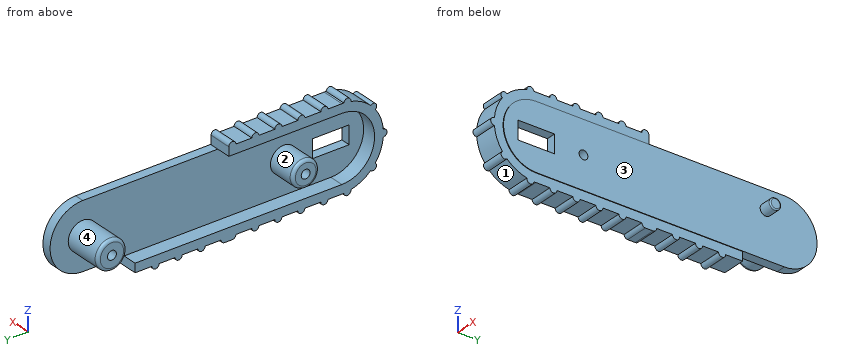
from build123d import *

# Parameters (mm, degrees)
PAD098_DEPTH            = 1.6
PAD099_DEPTH            = 4.05
POCKET093_DEPTH         = 0.1
SKETCH189_R             = 0.75
SKETCH189_W             = 6
SKETCH189_H             = 3
POCKET094_DEPTH         = 1.6
PAD100_DEPTH            = 3.95
SKETCH191_R             = 2.25
PAD101_DEPTH            = 4.9
SKETCH192_R             = 0.75
POCKET095_DEPTH         = 4.9
SKETCH193_R             = 2.475
PAD102_DEPTH            = 6.5
SKETCH194_R             = 0.75
POCKET096_DEPTH         = 6.5
FILLET041_R             = 0.5
SKETCH195_R             = 0.95
PAD103_DEPTH            = 2.2
FILLET042_R             = 0.2
SKETCH355_W             = 6.2
SKETCH355_H             = 3.1
POCKET171_DEPTH         = 5
BODY015_ROLL_ANGLE      = -90
BODY015_PLACEMENT_ANGLE = 90


with BuildPart() as part:
    # Sketch187 → Pad098 (new body)
    with BuildSketch(Plane.XY):
        with BuildLine():
            Line((0, 5.55), (42.05, 5.55))
            ThreePointArc((42.049962, -5.55), (47.599981, -1.9e-05), (42.05, 5.55))
            Line((42.049962, -5.55), (0, -5.55))
            ThreePointArc((0, 5.55), (-5.55, 0), (0, -5.55))
        make_face()
    extrude(amount=PAD098_DEPTH)

    # Sketch188 (on Face5 of Pad098) → Pad099 (join)
    with BuildSketch(Plane(origin=(0, 0, 0), x_dir=(1, 0, 0), z_dir=(0, 0, -1))):
        with BuildLine():
            Line((19.17, 5.55), (0, 5.55))
            ThreePointArc((0, 5.55), (-5.55, 0), (0, -5.55))
            Line((0, -5.55), (35.05, -5.55))
            Line((35.05, -5.55), (35.05, -7.05))
            Line((0, -7.05), (35.05, -7.05))
            ThreePointArc((0, 7.05), (-7.05, 0), (0, -7.05))
            Line((19.17, 7.05), (0, 7.05))
            Line((19.17, 5.55), (19.17, 7.05))
        make_face()
    extrude(amount=-PAD099_DEPTH)

    # Sketch188 (on Face5 of Pad098) → Pocket093 (cut)
    with BuildSketch(Plane(origin=(0, 0, 0), x_dir=(1, 0, 0), z_dir=(0, 0, -1))):
        with BuildLine():
            Line((19.17, 5.55), (0, 5.55))
            ThreePointArc((0, 5.55), (-5.55, 0), (0, -5.55))
            Line((0, -5.55), (35.05, -5.55))
            Line((35.05, -5.55), (35.05, -7.05))
            Line((0, -7.05), (35.05, -7.05))
            ThreePointArc((0, 7.05), (-7.05, 0), (0, -7.05))
            Line((19.17, 7.05), (0, 7.05))
            Line((19.17, 5.55), (19.17, 7.05))
        make_face()
    extrude(amount=-POCKET093_DEPTH, mode=Mode.SUBTRACT)

    # Sketch189 (on Face1 of Pocket093) → Pocket094 (cut)
    with BuildSketch(Plane(origin=(0, 0, 0), x_dir=(1, 0, 0), z_dir=(0, 0, -1))):
        with Locations((8, 0)):
            Circle(SKETCH189_R)
        Rectangle(SKETCH189_W, SKETCH189_H)
    extrude(amount=-POCKET094_DEPTH, mode=Mode.SUBTRACT)

    # Sketch190 (on Face11 of Pocket094) → Pad100 (join)
    with BuildSketch(Plane(origin=(0, 0, 0.1), x_dir=(1, 0, 0), z_dir=(0, 0, -1))):
        with BuildLine():
            ThreePointArc((19.17, 7.05), (18.57, 7.65), (17.97, 7.05))
            Line((19.17, 7.05), (17.97, 7.05))
        make_face()
        with BuildLine():
            ThreePointArc((15.27, 7.05), (14.67, 7.65), (14.07, 7.05))
            Line((15.27, 7.05), (14.07, 7.05))
        make_face()
        with BuildLine():
            ThreePointArc((11.37, 7.05), (10.77, 7.65), (10.17, 7.05))
            Line((11.37, 7.05), (10.17, 7.05))
        make_face()
        with BuildLine():
            ThreePointArc((7.47, 7.05), (6.87, 7.65), (6.27, 7.05))
            Line((7.47, 7.05), (6.27, 7.05))
        make_face()
        with BuildLine():
            ThreePointArc((3.57, 7.05), (2.97, 7.65), (2.37, 7.05))
            Line((3.57, 7.05), (2.37, 7.05))
        make_face()
        with BuildLine():
            ThreePointArc((-0.33, 7.042272), (-1.006549, 7.583492), (-1.51849, 6.884525))
            Line((-0.33, 7.042272), (-1.51849, 6.884525))
        make_face()
        with BuildLine():
            ThreePointArc((-4.890151, 5.078279), (-5.755669, 5.039323), (-5.679917, 4.176247))
            Line((-4.890151, 5.078279), (-5.679917, 4.176247))
        make_face()
        with BuildLine():
            ThreePointArc((-7.024468, 0.599457), (-7.65, 0), (-7.024468, -0.599457))
            Line((-7.024468, 0.599457), (-7.024468, -0.599457))
        make_face()
        with BuildLine():
            ThreePointArc((-5.677552, -4.179462), (-5.733191, -5.026164), (-4.886489, -5.081803))
            Line((-4.886489, -5.081803), (-5.677552, -4.179462))
        make_face()
        with BuildLine():
            ThreePointArc((-1.513526, -6.885618), (-1.001082, -7.584216), (-0.324923, -7.042508))
            Line((-0.324923, -7.042508), (-1.513526, -6.885618))
        make_face()
        with BuildLine():
            ThreePointArc((2.375077, -7.05), (2.975077, -7.65), (3.575077, -7.05))
            Line((3.575077, -7.05), (2.375077, -7.05))
        make_face()
        with BuildLine():
            ThreePointArc((6.275077, -7.05), (6.875077, -7.65), (7.475077, -7.05))
            Line((7.475077, -7.05), (6.275077, -7.05))
        make_face()
        with BuildLine():
            ThreePointArc((10.175077, -7.05), (10.775077, -7.65), (11.375077, -7.05))
            Line((11.375077, -7.05), (10.175077, -7.05))
        make_face()
        with BuildLine():
            ThreePointArc((14.075077, -7.05), (14.675077, -7.65), (15.275077, -7.05))
            Line((15.275077, -7.05), (14.075077, -7.05))
        make_face()
        with BuildLine():
            ThreePointArc((23.175077, -7.05), (23.775077, -7.65), (24.375077, -7.05))
            Line((24.375077, -7.05), (23.175077, -7.05))
        make_face()
        with BuildLine():
            ThreePointArc((27.075077, -7.05), (27.675077, -7.65), (28.275077, -7.05))
            Line((28.275077, -7.05), (27.075077, -7.05))
        make_face()
        with BuildLine():
            ThreePointArc((30.975077, -7.05), (31.575077, -7.65), (32.175077, -7.05))
            Line((32.175077, -7.05), (30.975077, -7.05))
        make_face()
        with BuildLine():
            ThreePointArc((17.975077, -7.05), (18.150813, -7.474264), (18.575077, -7.65))
            Line((19.875077, -7.65), (18.575077, -7.65))
            ThreePointArc((19.875077, -7.65), (20.299341, -7.474264), (20.475077, -7.05))
            Line((20.475077, -7.05), (17.975077, -7.05))
        make_face()
    extrude(amount=-PAD100_DEPTH)

    # Sketch191 (on Face12 of Pad100) → Pad101 (join)
    with BuildSketch(Plane.XY.offset(1.6)):
        with Locations((8, 0)):
            Circle(SKETCH191_R)
    extrude(amount=PAD101_DEPTH)

    # Sketch192 (on Face61 of Pad101) → Pocket095 (cut)
    with BuildSketch(Plane.XY.offset(6.5)):
        with Locations((8, 0)):
            Circle(SKETCH192_R)
    extrude(amount=-POCKET095_DEPTH, mode=Mode.SUBTRACT)

    # Sketch193 (on Face12 of Pocket095) → Pad102 (join)
    with BuildSketch(Plane.XY.offset(1.6)):
        with Locations((42.049981, 0)):
            Circle(SKETCH193_R)
    extrude(amount=PAD102_DEPTH)

    # Sketch194 (on Face62 of Pad102) → Pocket096 (cut)
    with BuildSketch(Plane.XY.offset(8.1)):
        with Locations((42.049981, 0)):
            Circle(SKETCH194_R)
    extrude(amount=-POCKET096_DEPTH, mode=Mode.SUBTRACT)

    # Fillet041
    fillet041_edges = [part.edges().sort_by_distance(p)[0] for p in [
        (39.574981, 0, 8.1),
        (5.75, 0, 6.5),
    ]]
    fillet(fillet041_edges, radius=FILLET041_R)

    # Sketch195 (on Face5 of Fillet041) → Pad103 (join)
    with BuildSketch(Plane(origin=(0, 0, 0), x_dir=(1, 0, 0), z_dir=(0, 0, -1))):
        with Locations((38.899981, 2.2)):
            Circle(SKETCH195_R)
    extrude(amount=PAD103_DEPTH)

    # Fillet042
    fillet042_edges = [part.edges().sort_by_distance(p)[0] for p in [
        (37.949981, -2.2, -2.2),
    ]]
    fillet(fillet042_edges, radius=FILLET042_R)

    # Sketch355 (on Face16 of Fillet042) → Pocket171 (cut)
    with BuildSketch(Plane.XY.offset(1.6)):
        Rectangle(SKETCH355_W, SKETCH355_H)
    extrude(amount=-POCKET171_DEPTH, mode=Mode.SUBTRACT)


with BuildPart() as part_1:
    # Body015 roll: moved
    add(part.part.rotate(Axis((0, 0, 0), (1, 0, 0)), BODY015_ROLL_ANGLE))


with BuildPart() as part_2:
    # Body015 placement: moved
    add(part_1.part.moved(Location((27.8, -51, -6.5))).rotate(Axis((27.8, -51, -6.5), (0, 0, 1)), BODY015_PLACEMENT_ANGLE))


solid = part_2.part
The model under review builds one solid part; all positions refer to its coordinate system, in mm. Face numbers are marked on the shaded views. Coordinates: 2 decimals unless noted, no trailing zeros. Order: outer loops, then holes, each group sorted by start corner. A loop starts at its lowest first (then second) coordinate and runs counter-clockwise, first axis right, second up. Notation, with made-up numbers: (22, -17) -> (34, -17) arc R12 ccw to (34, -8) -> close; hole circle Ø1 at (42.5, 81.5). An arc over 180 degrees is marked (long way). Answer in a Markdown table with one row per item.
(1) The part is to be moulded in two halves that separate along Z. For the marked faces 1, 2, 3 and 4, say which applies: +Z half, -Z half, draft (parallel to the pull), parting line (faces both ways), or undercut.
Answers:
| item | result |
|---|---|
| face 1 | -Z half |
| face 2 | undercut |
| face 3 | draft |
| face 4 | parting line |
(2) Consider section D-D (y = -26). Write out the cut boundary in (x, z), plus the area to 3 significant figures.
Answers:
| item | result |
|---|---|
| outline | (23.75, -13.55) -> (27.7, -13.55) -> (27.7, -12.05) -> (27.8, -12.05) -> (27.8, -0.95) -> (26.2, -0.95) -> (26.2, -12.05) -> (23.75, -12.05) -> close |
| area | 23.7 mm² |
(3) Insertion check: pin 1 (0.5 mm diameter, centred on x = 25.5, z = -13, fed in from +Y); pin 2 (0.5 mm diameter, centred on x = 26, z = 0, fed in from +Y); pin 3 (0.8 mm diameter, centred on x = 27, z = -7, fed in from +Y); pin 4 (1.4 mm diameter, centred on x = 25.5, y = -38, fed in from +Z). Each pin has a flat end and moves straight along its axis. Give the tip position at first contact, or say it passes through.
Answers:
| item | result |
|---|---|
| pin 1 | y = -15.95 |
| pin 2 | y = -31.83 |
| pin 3 | y = -3.4 |
| pin 4 | z = 0.55 |
(4) Consider section A-A (y = -43). Write out the cut boundary in (x, z).
Answers:
| item | result |
|---|---|
| outline | (21.3, -8.25) arc R0.5 ccw to (21.8, -8.75) -> (26.2, -8.75) -> (26.2, -12.05) -> (23.75, -12.05) -> (23.75, -13.55) -> (27.7, -13.55) -> (27.7, -12.05) -> (27.8, -12.05) -> (27.8, -7.25) -> (21.3, -7.25) -> close; (21.3, -5.75) -> (27.8, -5.75) -> (27.8, -0.95) -> (27.7, -0.95) -> (27.7, 0.55) -> (23.75, 0.55) -> (23.75, -0.95) -> (26.2, -0.95) -> (26.2, -4.25) -> (21.8, -4.25) arc R0.5 ccw to (21.3, -4.75) -> close |
(5) Wall thickness on line 1 along Y through (x, z) = (24.25, -6.5); line 2 along Z through (x, y) = (26.75, -43); line 3 along Z through (x, y) = (24.75, -43): over which ranges is each line inside the solid? List them lowest first.
Answers:
| item | result |
|---|---|
| line 1 | -58.65 to -56.55, -45.25 to -43.75, -42.25 to -40.75, -11.43 to -9.7, -8.2 to -6.48 |
| line 2 | -13.55 to -7.25, -5.75 to 0.55 |
| line 3 | -13.55 to -12.05, -8.75 to -7.25, -5.75 to -4.25, -0.95 to 0.55 |
(6) Consider section B-B (z = -6.5). State how many separate pieces and enclosed holes the cut face has, plus the area to 3 significant figures.
Answers:
| item | result |
|---|---|
| separate pieces | 3 |
| enclosed holes | 0 |
| area | 118 mm² |
